from build123d import *

# Parameters (mm, degrees)
F0_W     = 53.1371047842
F0_H     = 24.2517590523
F1_DEPTH = 12.5
F2_W     = 17.8484022617
F2_H     = 6.8188142031
F3_DEPTH = 25
F4_SIZE  = 5
F5_R     = 3


with BuildPart() as f1:
    # F0 (on Front) → F1 (new body, symmetric)
    with BuildSketch(Plane.XZ):
        Rectangle(F0_W, F0_H)
    extrude(amount=F1_DEPTH, both=True)

    # F2 (on face) → F3 (cut)
    with BuildSketch(Plane.XZ.offset(12.5)):
        with Locations((-0.3203526139, 3.4094071016)):
            Rectangle(F2_W, F2_H)
    extrude(amount=-F3_DEPTH, mode=Mode.SUBTRACT)

    # F4
    f4_edges = [f1.edges().sort_by_distance(p)[0] for p in [
        (-26.568552, 0, 12.12588),
        (26.568552, 0, 12.12588),
    ]]
    chamfer(f4_edges, length=F4_SIZE)

    # F5
    f5_edges = [f1.edges().sort_by_distance(p)[0] for p in [
        (0, -12.5, 12.12588),
        (0, 12.5, 12.12588),
        (-21.568552, 0, 12.12588),
        (21.568552, 0, 12.12588),
    ]]
    fillet(f5_edges, radius=F5_R)


solid = f1.part
Check sheet for the modelled part. Datum: model origin and axes. Units: mm. A direction names the side the tool comes from. Round coordinates to 2 decimals unless told otherwise and drop trailing zeros. Order: outer loops, then holes, each group sorted by start corner. A loop starts at its lowest first (then second) coordinate and runs counter-clockwise, first axis right, second up.
Q1. Cross-section at A-A, the plane x = -3. Enter the section's corners in (y, z).
Filled sheet:
outline: (-12.5, -12.13) - (12.5, -12.13) - (12.5, 0) - (-12.5, 0) - close; (-12.5, 6.82) - (12.5, 6.82) - (12.5, 9.13) arc R3 ccw to (9.5, 12.13) - (-9.5, 12.13) arc R3 ccw to (-12.5, 9.13) - close
Q2. Scan lines: L1, parallel to X at y = -10.25, z = 2.5; L2, parallel to Z at x = -3, y = -1; L3, parallel to Z at x = 24.5, y = 6.25. Record each from-to range of solid material in increasing order.
Filled sheet:
L1: x = -26.57 to -9.24, 8.6 to 26.57
L2: z = -12.13 to 0, 6.82 to 12.13
L3: z = -12.13 to 9.19
Q3. Draft check along Z on faces 1 (the face through (0, -12.5, -1)), 2 (the face through (0.344, 11.645, 11.224)), 3 (the face through (-9.245, 0, 3)), 4 (the face through (0, 0, -12.126)). Enter one of: pulls with the +Z half, pulls with the -Z half, needs draft (parallel to the pull), parting line crosses it, or undercut.
Filled sheet:
face 1: needs draft
face 2: pulls with the +Z half
face 3: undercut
face 4: pulls with the -Z half
Q4. Set-up check for faces 5 (the face through (8.604, 0, 3)), 6 (the face through (-26.569, 0, -3)): record each of +Z, -Z, +X, -X, +Y, -Y from which the full face is reachable in a straight line by a thin tool's end or side.
Filled sheet:
face 5: +Y, -Y
face 6: +Z, -Z, -X, +Y, -Y
Q5. Cross-section at D-D, the plane z = 9.75. Enter the section's corners in (x, y).
Filled sheet:
outline: (-23.94, -12.43) - (23.94, -12.43) - (23.94, 12.43) - (-23.94, 12.43) - close
Q6. Cross-section at C-C, the plane z = 2.75. Enter the section's corners in (x, y), plus the area to 3 significant figures.
Filled sheet:
outline: (-26.57, -12.5) - (-9.24, -12.5) - (-9.24, 12.5) - (-26.57, 12.5) - close; (8.6, -12.5) - (26.57, -12.5) - (26.57, 12.5) - (8.6, 12.5) - close
area: 882 mm2
Q7. Cross-section at B-B, the plane y = 5.25. Enter the section's corners in (x, z), plus the area to 3 significant figures.
Filled sheet:
outline: (-26.57, -12.13) - (26.57, -12.13) - (26.57, 7.13) - (22.45, 11.25) arc R3 ccw to (20.33, 12.13) - (-20.33, 12.13) arc R3 ccw to (-22.45, 11.25) - (-26.57, 7.13) - close; hole (-9.24, 0) - (8.6, 0) - (8.6, 6.82) - (-9.24, 6.82) - close
area: 1,140 mm2
